Input: part model. Units: mm. Frame: model coordinates. Face numbers are marked on the shaded views. A direction names the side the tool comes from. Give positions to 0.01 mm unless a question says otherwise; leave off trailing zeros. Loops run counter-clockwise (first coordinate to the right, second up) from the corner with the lowest first, then second, coordinate; pieces in that order, holes last. Notation, with made-up numbers: (-14.75, 81) -> (-3.75, 81) arc R27 ccw to (-3.75, 106) -> close; hole circle Ø10 at (13.5, 63). An arc over 180 degrees is marked (long way). Answer as a JSON object with one key per item and string values. Group by question number.
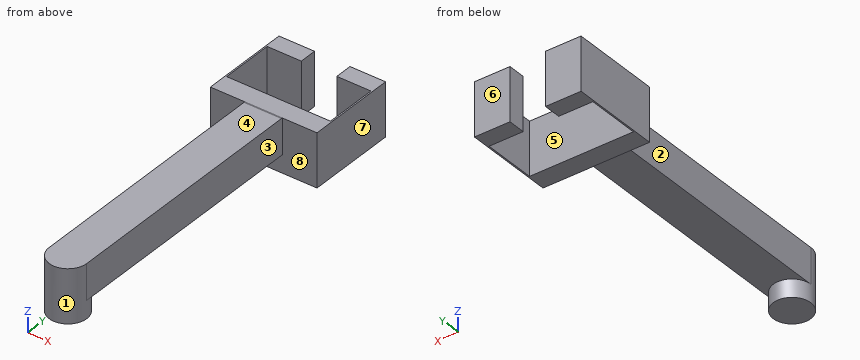
```python
from build123d import *

# Parameters (mm, degrees)
SKETCH2_R           = 13.4112
BOSS_EXTRUDE1_DEPTH = 38.1
SKETCH5_W           = 26.8224
SKETCH5_H           = 184.15
BOSS_EXTRUDE2_DEPTH = 25.4
SKETCH8_W           = 76.2
SKETCH8_H           = 38.1
BOSS_EXTRUDE3_DEPTH = 13.97
SKETCH9_W           = 1.016
SKETCH9_H           = 38.1
BOSS_EXTRUDE4_DEPTH = 38.1
SKETCH10_W          = 25.4
SKETCH10_H          = 38.1
BOSS_EXTRUDE5_DEPTH = 12.446
FILLET1_R           = 3.81


with BuildPart() as part:
    # Sketch2 → Boss-Extrude1 (new body)
    with BuildSketch(Plane.XY):
        with Locations(Location((0, 0, 0), (0, 0, 180))):
            Circle(SKETCH2_R)
    extrude(amount=BOSS_EXTRUDE1_DEPTH)

    # Sketch5 → Boss-Extrude2 (add)
    with BuildSketch(Plane.XY.offset(38.1)):
        with Locations((0, 92.075)):
            Rectangle(SKETCH5_W, SKETCH5_H)
    extrude(amount=-BOSS_EXTRUDE2_DEPTH)

    # Sketch8 → Boss-Extrude3 (add)
    with BuildSketch(Plane(origin=(0, 184.15, 0), x_dir=(1, 0, 0), z_dir=(0, 1, 0))):
        with Locations((0, -18.948214994)):
            Rectangle(SKETCH8_W, SKETCH8_H)
    extrude(amount=BOSS_EXTRUDE3_DEPTH)

    # Sketch9 → Boss-Extrude4 (add)
    with BuildSketch(Plane(origin=(0, 198.12, 0), x_dir=(1, 0, 0), z_dir=(0, 1, 0))):
        with Locations((-37.592, -18.948214994)):
            Rectangle(SKETCH9_W, SKETCH9_H)
        with Locations((37.592, -18.948214994)):
            Rectangle(SKETCH9_W, SKETCH9_H)
    extrude(amount=BOSS_EXTRUDE4_DEPTH)

    # Sketch10 → Boss-Extrude5 (add)
    with BuildSketch(Plane(origin=(0, 236.22, 0), x_dir=(1, 0, 0), z_dir=(0, 1, 0))):
        with Locations((-25.4, -18.948214994)):
            Rectangle(SKETCH10_W, SKETCH10_H)
        with Locations((25.4, -18.948214994)):
            Rectangle(SKETCH10_W, SKETCH10_H)
    extrude(amount=BOSS_EXTRUDE5_DEPTH)

    # Fillet1
    # the kernel refuses this fillet: 3.81 mm, written as the material it takes off along each edge
    with BuildSketch(Plane(origin=(15.598152153, 184.15, 38.1), x_dir=(0, 0, -1), z_dir=(-1, 0, 0))) as fillet1_piece_1:
        with BuildLine():
            CenterArc((3.81, 0.874780861), FILLET1_R, 180, 13.273598337)
            Line((0, 0.874780861), (-0.0762, 0.874780861))
            Line((-0.0762, 0.874780861), (-0.0762, 0))
            Line((-0.0762, 0), (0, -0.0762))
            ThreePointArc((0, -0.0762), (0.050892503, -0.0762), (0.027620706, -0.017495617))
            Line((0.027620706, -0.017495617), (0.101785006, 0))
        make_face()
    extrude(amount=31.196304306, mode=Mode.SUBTRACT)


solid = part.part
```
Q1. Ray query, probe 1 along Y at (x, z) = (-35, 10); probe 2 along X at (y, z) = (221.5, 3); probe 3 along X at (y, z) = (-0.5, 24). Return the intervals inside material, ascending.
Q2. Section B-B on z = 6. Return the cut outline in (x, y).
Q3. Pull-direction query (Y, two-part tool) for the marked faces 6, 7 and 8; classes: +Y half, -Y half, draft (parallel to the pull), parting line (faces both ways), or undercut.
Q4. Section D-D on x = 0. Return the cut outline in (y, z).
Q5. Set-up query: the marked faces 1, 2, 3, 4 and 5. Return all of +Z, -Z, +X, -X, +Y, -Y with unobstructed straight access to the full face (end or side cutting, diameter ignored); none if empty.
Q6. Pin query (flat end, axial travel): pin 1 Ø1 at (x, z) = (3, 10.5) entering from +Y; pin 2 Ø2 at (x, y) = (-15.5, 139) entering from -Z; pin 3 Ø13.5 at (x, y) = (3.5, 85) entering from -Z; pin 4 Ø3 at (x, z) = (-12.5, 18.5) entering from -Y. Return the tip coordinate at first contact, or that it passes through.
Q7. Section A-A on x = -30. Return the cut outline in (y, z).
Q8. Section C-C on y = 209. Return the cut outline in (x, z).
Numbers:
{
 "1": {"probe 1": "y = 184.15 to 198.12, 236.22 to 248.67", "probe 2": "x = -38.1 to -37.08, 37.08 to 38.1", "probe 3": "x = -13.4 to 13.4"},
 "2": {"outline": "(-38.1, 184.15) -> (38.1, 184.15) -> (38.1, 248.67) -> (12.7, 248.67) -> (12.7, 236.22) -> (37.08, 236.22) -> (37.08, 198.12) -> (-37.08, 198.12) -> (-37.08, 236.22) -> (-12.7, 236.22) -> (-12.7, 248.67) -> (-38.1, 248.67) -> close; circle Ø26.82 at (0, 0)"},
 "3": {"face 6": "+Y half", "face 7": "draft", "face 8": "undercut"},
 "4": {"outline": "(-13.41, 0) -> (13.41, 0) -> (13.41, 12.7) -> (184.15, 12.7) -> (184.15, -0.1) -> (198.12, -0.1) -> (198.12, 38) -> (184.15, 38) arc R3.81 ccw to (183.28, 38.1) -> (-13.41, 38.1) -> close"},
 "5": {"face 1": "-Z", "face 2": "+Z, -Z, -X, -Y", "face 3": "+Z, -Z, +X, -Y", "face 4": "+Z, +X, -X, +Y, -Y", "face 5": "+Z, -Z"},
 "6": {"pin 1": "stops at y = 198.12", "pin 2": "passes through", "pin 3": "stops at z = 12.7", "pin 4": "stops at y = -7.67"},
 "7": {"outline": "(184.15, -0.1) -> (198.12, -0.1) -> (198.12, 38) -> (184.15, 38) -> close; (236.22, -0.1) -> (248.67, -0.1) -> (248.67, 38) -> (236.22, 38) -> close"},
 "8": {"outline": "(-38.1, -0.1) -> (-37.08, -0.1) -> (-37.08, 38) -> (-38.1, 38) -> close; (37.08, -0.1) -> (38.1, -0.1) -> (38.1, 38) -> (37.08, 38) -> close"}
}
